Here's how the part is built. I have some questions about the finished solid (model axes, mm). Round coordinates to 2 decimals unless told otherwise and drop trailing zeros. Loops run counter-clockwise (first coordinate to the right, second up) from the corner with the lowest first, then second, coordinate; pieces in that order, holes last. Notation, with made-up numbers: M 8,72 L 27,72 A14 cw 27,84 Z; hole C -17.75,23 d4. An arc over 180 degrees is marked long. Answer as a JSON object with one key per item and string values.
Autodesk Inventor part; units mm, degrees
ref_plane "YZ Plane" through (0, 0, 0) normal (1, 0, 0) x (0, 1, 0)
ref_plane "XZ Plane" through (0, 0, 0) normal (0, 1, 0) x (-1, 0, 0)
ref_plane "XY Plane" through (0, 0, 0) normal (0, 0, 1) x (1, 0, 0)
sketch "Sketch1" plane through (0, 0, 0) normal (0, 1, 0) x (-1, 0, 0)
  line L0 (0, 0) -> (-133.35, 0)
  line L1 (-133.35, 0) -> (-133.35, 25.4)
  line L2 (-133.35, 25.4) -> (0, 25.4)
  line L3 (0, 25.4) -> (0, 0)
  line L4 (-133.35, 25.4) -> (-143.871, 0)
  line L5 (-133.35, 25.4) -> (-105.8572, 25.4) construction
  line L6 (-133.35, 25.4) -> (-151.3105, 7.4395)
  line L7 (-133.35, 25.4) -> (-107.95, 25.4) construction
  line L8 (-151.3105, 7.4395) -> (-143.871, 0)
  line L9 (-133.35, 25.4) -> (-151.3105, 7.4395)
  line L10 (-151.3105, 7.4395) -> (-318.9899, 175.1188)
  line L11 (-318.9899, 175.1188) -> (-301.0293, 193.0793)
  line L12 (-301.0293, 193.0793) -> (-133.35, 25.4)
  circle A0 centre (-12.7, 12.7) radius 6.35
  line L13 (-318.9899, 175.1188) -> (-511.6743, 175.1188)
  line L14 (-511.6743, 175.1188) -> (-511.6743, 200.5188)
  line L15 (-511.6743, 200.5188) -> (-318.9899, 200.5188)
  line L16 (-318.9899, 200.5188) -> (-318.9899, 175.1188)
  line L17 (-318.9899, 175.1188) -> (-308.4688, 200.5188)
  line L18 (-308.4688, 200.5188) -> (-318.9899, 200.5188)
  line L19 (-308.4688, 200.5188) -> (-301.0293, 193.0793)
  line L20 (-133.35, 0) -> (-143.871, 0)
  dimension "d0" = 133.35
  dimension "d1" = 25.4
  dimension "d2" = 112.5
  dimension "d3" = 25.4
  dimension "d4" = 135
  dimension "d5" = 237.1344
  dimension "d6" = 12.7
  dimension "d7" = 192.6844
  dimension "d8" = 25.4
extrude "Extrusion1" add sketch "Sketch1" along normal blind 6.35
sketch "Sketch2" plane through (511.6743, 0, 200.5188) normal (1, 0, 0) x (0, 0, -1)
  line L0 (0, 6.35) -> (25.4, 6.35)
  line L1 (25.4, 0) -> (0, 0)
  line L2 (0, 0) -> (0, 25.4)
  line L3 (0, 25.4) -> (25.4, 25.4)
  line L4 (25.4, 25.4) -> (25.4, 0)
  point P0 (200.5188, 0)
  dimension "d15" = 25.4
  dimension "d16" = 25.4
extrude "Extrusion2" add sketch "Sketch2" along normal blind 1.5875
sketch "Sketch3" plane through (0, 0, 0) normal (-1, 0, 0) x (0, 0, 1)
  line L0 (0, 0) -> (25.4, 0)
  line L1 (25.4, 0) -> (25.4, 6.35)
  line L2 (0, 6.35) -> (25.4, 6.35)
  line L3 (0, 0) -> (0, 6.35)
extrude "Extrusion3" add sketch "Sketch3" along normal blind 44.45
sketch "Sketch5" plane through (0, 6.35, 0) normal (0, 1, 0) x (1, 0, 0)
  circle A0 centre (12.7, -12.7) radius 6.35
  line L0 (511.6743, -175.1188) -> (318.9899, -175.1188)
  line L1 (12.7, -12.7) -> (12.7, -6.35)
  line L2 (16.3662, -6.35) -> (20.0323, -12.7)
  line L3 (20.0323, -12.7) -> (16.3662, -19.05)
  line L4 (16.3662, -19.05) -> (9.0338, -19.05)
  line L5 (9.0338, -19.05) -> (5.3677, -12.7)
  line L6 (5.3677, -12.7) -> (9.0338, -6.35)
  line L7 (9.0338, -6.35) -> (16.3662, -6.35)
  point P0 (0, 0)
extrude "Extrusion5" cut sketch "Sketch5" against normal blind 6.35 contours A0 L2 L3 | A0 L7 L2 | L3 L4 A0 | A0 L6 L7 | L4 L5 A0 | A0 L5 L6
sketch "Sketch7" plane through (0, 6.35, 0) normal (0, 1, 0) x (1, 0, 0)
  line L0 (-44.45, -25.4) -> (-44.45, 0)
  line L1 (511.6743, -175.1188) -> (318.9899, -175.1188)
  line L2 (-44.45, -12.7) -> (12.7, -12.7)
  line L3 (12.7, -12.7) -> (-25.4, -12.7)
  line L4 (12.7, -12.7) -> (50.8, -12.7) construction
  line L5 (-25.4, -12.7) -> (50.8, -12.7)
  circle A0 centre (-25.4, -12.7) radius 3.175
  circle A1 centre (50.8, -12.7) radius 3.175
  point P0 (0, 0)
  dimension "d31" = 38.1
  dimension "d32" = 180
  dimension "d33" = 76.2
  dimension "d34" = 0
  dimension "d35" = 6.35
  dimension "d36" = 6.35
extrude "Extrusion7" cut sketch "Sketch7" against normal blind 25.4
sketch "Sketch8" plane through (0, 6.35, 0) normal (0, 1, 0) x (1, 0, 0)
  circle A0 centre (-25.4, -12.7) radius 3.175
  circle A1 centre (50.8, -12.7) radius 3.175
  line L0 (-44.45, 0) -> (0, 0)
  line L1 (0, 0) -> (0, -25.4)
  line L2 (0, -25.4) -> (-44.45, -25.4)
  line L3 (-44.45, -25.4) -> (-44.45, 0)
  line L4 (0, -12.7) -> (12.7, -12.7)
  line L5 (12.7, -12.7) -> (50.8, -12.7)
  line L6 (50.8, -12.7) -> (88.9, -12.7)
  circle A2 centre (88.9, -12.7) radius 3.175
  dimension "d39" = 44.45
  dimension "d40" = 25.4
  dimension "d41" = 38.1
  dimension "d42" = 180
  dimension "d43" = 6.35
extrude "Extrusion8" cut sketch "Sketch8" against normal blind 25.4 contours L1 L2 L3 L0 | A2
sketch "Sketch9" plane through (0, 6.35, 0) normal (-1, 0, 0) x (0, 0, 1)
  line L0 (25.4, -6.35) -> (0, -6.35)
  line L1 (25.4, 0) -> (25.4, -6.35)
  line L2 (0, 0) -> (25.4, 0)
  line L3 (0, -6.35) -> (0, 0)
extrude "Extrusion9" add sketch "Sketch9" along normal blind 6.35
sketch "Sketch10" plane through (0, 6.35, 0) normal (0, 1, 0) x (1, 0, 0)
  line L0 (-6.35, -25.4) -> (-6.35, 0)
  line L1 (5.3677, -12.7) -> (9.0338, -6.35)
  line L2 (9.0338, -6.35) -> (16.3662, -6.35)
  line L3 (16.3662, -6.35) -> (20.0323, -12.7)
  line L4 (20.0323, -12.7) -> (16.3662, -19.05)
  line L5 (16.3662, -19.05) -> (9.0338, -19.05)
  line L6 (9.0338, -19.05) -> (5.3677, -12.7)
  line L7 (-6.35, -12.7) -> (12.7, -12.7)
  line L8 (12.7, -12.7) -> (6.35, -12.7)
  line L9 (12.7, -12.7) -> (19.05, -12.7) construction
  line L10 (6.35, -12.7) -> (9.525, -7.2007)
  line L11 (9.525, -7.2007) -> (15.875, -7.2007)
  line L12 (15.875, -7.2007) -> (19.05, -12.7)
  line L13 (19.05, -12.7) -> (15.875, -18.1993)
  line L14 (15.875, -18.1993) -> (9.525, -18.1993)
  line L15 (9.525, -18.1993) -> (6.35, -12.7)
  point P0 (0, 0)
  dimension "d48" = 6.35
  dimension "d49" = 180
extrude "Extrusion10" add sketch "Sketch10" against normal blind 6.35
properties part number "Z-PickupArm-L"
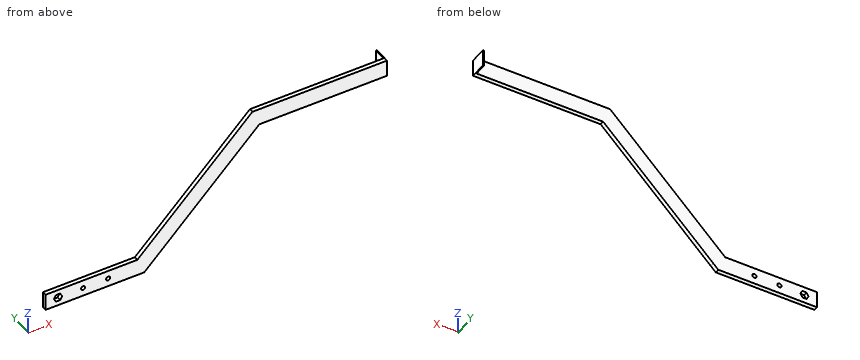
Item 1: If I drill on L1, parallel to Z at x = 50.8, y = 4.5 (3 decimals); L2, parallel to X at y = 3, z = 12.7 (3 decimals); L3, parallel to Y at x = 288, z = 161, over which ranges is the centre line in solid material (lowest first)? Write a range as from..to.
Solution:
{"L1": "z = 0..9.525, 15.875..25.4", "L2": "x = -6.35..6.35, 19.05..47.625, 53.975..85.725, 92.075..156.571", "L3": "y = 0..6.35"}
Item 2: For P1, Ø8.5, axis at x = 88.9, z = 12.7, coming from the +Y side; P2, Ø5.5, axis at y = 20.5, z = 185.5, coming from the -X side; P3, Ø1.9, axis at x = 91.5, y = 4, coming from the +Z side, each with a flat end and sliding along its axis, tell me the tip position at first contact or that it passes through.
Solution:
{"P1": "stops at y = 6.35", "P2": "stops at x = 511.67", "P3": "stops at z = 25.4"}
Item 3: I want a section at A-A on x = 323.5. List the corners of the cut face in (y, z) for me.
Solution:
{"outline": "M 0,175.12 L 6.35,175.12 L 6.35,200.52 L 0,200.52 Z"}
Item 4: I want a section at B-B on y = 18.75. List the corners of the cut face in (x, z) for me, plus the area to 3 significant figures.
Solution:
{"outline": "M 511.67,175.12 L 513.26,175.12 L 513.26,200.52 L 511.67,200.52 Z", "area": "40.3 mm2"}
